from build123d import *

# Parameters (mm, degrees)
F0_W      = 89.3173888326
F0_H      = 89.3173888326
F1_DEPTH  = 25
F3_DEPTH  = 10
F4_R      = 35
F5_DEPTH  = 25
F6_R      = 4
F7_T      = -1
F8_DEPTH  = 41.7
F9_R      = 1.5
F10_DEPTH = 3.8
F12_COUNT = 4


with BuildPart() as f1:
    # F0 (on Top) → F1 (new body)
    with BuildSketch(Plane.XY):
        Rectangle(F0_W, F0_H)
    extrude(amount=F1_DEPTH)

    # F2 (on face) → F3 (join)
    with BuildSketch(Plane.XY.offset(25)):
        Polygon((32.6586944163, 44.6586944163), (-32.6586944163, 44.6586944163), (-44.6586944163, 32.6586944163), (-44.6586944163, -32.6586944163), (-32.6586944163, -44.6586944163), (32.6586944163, -44.6586944163), (44.6586944163, -32.6586944163), (44.6586944163, 32.6586944163), align=None)
    extrude(amount=F3_DEPTH)

    # F4 (on face) → F5 (join)
    with BuildSketch(Plane.XY.offset(35)):
        Circle(F4_R)
    extrude(amount=F5_DEPTH)

    # F6
    f6_edges = [f1.edges().sort_by_distance(p)[0] for p in [
        (44.658694, 44.658694, 12.5),
        (44.658694, -44.658694, 12.5),
        (-44.658694, -44.658694, 12.5),
        (-44.658694, 44.658694, 12.5),
    ]]
    fillet(f6_edges, radius=F6_R)

    # F7
    f7_openings = [f1.faces().sort_by_distance(p)[0] for p in [
        (0, 0, 0),
    ]]
    offset(amount=F7_T, openings=f7_openings, kind=Kind.INTERSECTION)

    # F8 (cut): a face of the model
    f8_faces = [f1.faces().sort_by_distance(p)[0] for p in [
        (0, 0, 59),
    ]]
    extrude(f8_faces, amount=-F8_DEPTH, mode=Mode.SUBTRACT)


with BuildPart() as f10:
    # F9 (on face) → F10 (new body, symmetric)
    with BuildSketch(Plane.XY.offset(25)):
        with Locations((-40.6586944163, 40.6586944163)):
            Circle(F9_R)
    extrude(amount=F10_DEPTH, both=True)


with BuildPart() as f12_1:
    # F12: instance of F10
    add(f10.part.rotate(Axis((0, 0, 19.2969664931), (0, 0, 1)), 1 * 360 / F12_COUNT))


with BuildPart() as f12_2:
    # F12: instance of F10
    add(f10.part.rotate(Axis((0, 0, 19.2969664931), (0, 0, 1)), 2 * 360 / F12_COUNT))


with BuildPart() as f12_3:
    # F12: instance of F10
    add(f10.part.rotate(Axis((0, 0, 19.2969664931), (0, 0, 1)), 3 * 360 / F12_COUNT))


with BuildPart() as f1_1:
    add(f1.part)

    # F13: cut F10, F12_3, F12_2, F12_1
    add(f10.part, mode=Mode.SUBTRACT)
    add(f12_3.part, mode=Mode.SUBTRACT)
    add(f12_2.part, mode=Mode.SUBTRACT)
    add(f12_1.part, mode=Mode.SUBTRACT)


solid = f1_1.part
Build history of the part. All positions in model axes, mm. A direction names the side the tool comes from. Give positions to 0.01 mm unless a question says otherwise; leave off trailing zeros. Order: outer loops, then holes, each group sorted by start corner. A loop starts at its lowest first (then second) coordinate and runs counter-clockwise, first axis right, second up. Notation, with made-up numbers: M 69.5,89.5 L 81.5,89.5 A28 ccw 81.5,109.5 Z; hole C 84.25,-15 d6. An arc over 180 degrees is marked long. Use one line per item in the form item = value.
Q1. Slice it at D-D, the plane z = 56. Write the cut outline in (x, y).
Conclusion:
outline = C 0,0 d70; hole C 0,0 d68
Q2. Slice it at A-A, the plane y = 0. Write the cut outline in (x, z).
Conclusion:
outline = M -44.66,0 L -43.66,0 L -43.66,34 L -34,34 L -34,60 L -35,60 L -35,35 L -44.66,35 Z; M 34,34 L 43.66,34 L 43.66,0 L 44.66,0 L 44.66,35 L 35,35 L 35,60 L 34,60 Z
Q3. Wall check: probe 1 along X at (y, z) = (24, 15.5); probe 2 along Y at (x, z) = (0, 46.75); probe 3 along Y at (x, z) = (-4.5, 37). Give the ranges that are in metal, low to high.
Conclusion:
probe_1 = -44.66 to -43.66, 43.66 to 44.66
probe_2 = -35 to -34, 34 to 35
probe_3 = -34.71 to -33.7, 33.7 to 34.71
Q4. Slice it at C-C, the plane z = 10.5. Write the cut outline in (x, y), and give its area (3 significant figures).
Conclusion:
outline = M -44.66,-40.66 A4 ccw -40.66,-44.66 L 40.66,-44.66 A4 ccw 44.66,-40.66 L 44.66,40.66 A4 ccw 40.66,44.66 L -40.66,44.66 A4 ccw -44.66,40.66 Z; hole M -43.66,-40.66 A3 ccw -40.66,-43.66 L 40.66,-43.66 A3 ccw 43.66,-40.66 L 43.66,40.66 A3 ccw 40.66,43.66 L -40.66,43.66 A3 ccw -43.66,40.66 Z
area = 347 mm2
Q5. Pull direction Y, two halves, no side cores. Call faces 1 (the cylindrical face through (-39.75, -41.85, 24.51)), 2 (the flat face through (-1, 44.659, 17)), 3 (the flat face through (38.575, -38.743, 29.93)), 4 (the flat face through (-39, 40, 25)): released by +Y, released by -Y, zero draft, split by the parting line, or undercut.
Conclusion:
face_1 = undercut
face_2 = released by +Y
face_3 = released by -Y
face_4 = zero draft
Q6. Pin check, flat tips, straight feed: P1, Ø3.5, axis at x = 40.66, y = 40.66, coming from the -Z side; P2, Ø9.5, axis at x = -39.5, y = 36, coming from the +Z side; P3, Ø5.5, axis at x = 35.5, y = -35, coming from the -Z side; P4, Ø1.8, axis at x = 40.66, y = -40.66, coming from the +Z side. Stop position of each tip, or through.
Conclusion:
P1 = 24
P2 = 35
P3 = 34
P4 = through
Q7. Which spindle directions (+Z, -Z, +X, -X, +Y, -Y) get a long thin tool onto all of the face, cutting with end or side? Do faces 5 (the flat face through (-38.575, 38.743, 29.93)), 6 (the flat face through (-41, -43, 25)), 7 (the cylindrical face through (42.76, 42.8, 12.17)). Say none if no direction does.
Conclusion:
face_5 = +Z, -X, +Y
face_6 = +Z, -X, -Y
face_7 = -Z
